```python
from build123d import *

# Parameters (mm, degrees)
F0_W     = 32
F0_H     = 32
F1_DEPTH = 600
F3_D     = 14
F3_DEPTH = 45
F4_D     = 14
F4_DEPTH = 45
F6_D     = 5
F6_DEPTH = 5
F7_D     = 5
F7_DEPTH = 5


with BuildPart() as f1:
    # F0 (on Front) → F1 (new body)
    with BuildSketch(Plane.XZ):
        with BuildLine():
            Line((-15, -20), (15, -20))
            ThreePointArc((15, -20), (18.535534, -18.535534), (20, -15))
            Line((20, -15), (20, 15))
            ThreePointArc((20, 15), (18.535534, 18.535534), (15, 20))
            Line((15, 20), (-15, 20))
            ThreePointArc((-15, 20), (-18.535534, 18.535534), (-20, 15))
            Line((-20, 15), (-20, -15))
            ThreePointArc((-20, -15), (-18.535534, -18.535534), (-15, -20))
        make_face()
        Rectangle(F0_W, F0_H, mode=Mode.SUBTRACT)
    extrude(amount=F1_DEPTH)

    # F3
    with Locations(Plane.YZ.offset(20)):
        with Locations((-560, 0)):
            Hole(F3_D / 2, depth=F3_DEPTH)

    # F4
    with Locations(Plane.YZ.offset(20)):
        with Locations((-40, 0)):
            Hole(F4_D / 2, depth=F4_DEPTH)

    # F6
    with Locations(Plane(origin=(0, 0, -20), x_dir=(1, 0, 0), z_dir=(0, 0, -1))):
        with Locations((0, 525)):
            Hole(F6_D / 2, depth=F6_DEPTH)

    # F7
    with Locations(Plane(origin=(0, 0, -20), x_dir=(1, 0, 0), z_dir=(0, 0, -1))):
        with Locations((0, 75)):
            Hole(F7_D / 2, depth=F7_DEPTH)


solid = f1.part
```
Geometry check sheet. Reference: the model listing, model coordinates, mm. A direction names the side the tool comes from. Coordinates: 2 decimals unless noted, no trailing zeros. Order: outer loops, then holes, each group sorted by start corner. A loop starts at its lowest first (then second) coordinate and runs counter-clockwise, first axis right, second up. Notation, with made-up numbers: M 13.25,52.5 L 46.25,52.5 A14 ccw 46.25,61.5 Z; hole C 41.5,46.5 d3. An arc over 180 degrees is marked long. Answer as a JSON object with one key per item and string values.
Q1. Cross-section at A-A on y = -40. Record the cut outline in (x, z).
Results are:
{"outline": "M -20,-15 A5 ccw -15,-20 L 15,-20 A5 ccw 20,-15 L 20,-7 L 16,-7 L 16,-16 L -16,-16 L -16,-7 L -20,-7 Z; M -20,7 L -16,7 L -16,16 L 16,16 L 16,7 L 20,7 L 20,15 A5 ccw 15,20 L -15,20 A5 ccw -20,15 Z"}
Q2. Release check for a two-part mould opening along Z. For faces 1 (the flat face through (-18, 0, 0)), 2 (the flat face through (0, -296, -20)), 3 (the flat face through (0, -296, 20)), 4 (the cylindrical face through (-18.028, -566.677, 2.103)) record: released by +Z, released by -Z, zero draft, split by the parting line, or undercut.
Results are:
{"face 1": "zero draft", "face 2": "released by -Z", "face 3": "released by +Z", "face 4": "undercut"}
Q3. Scan lines: line 1 (Y direction, x = 0, z = -16.9); line 2 (Z direction, x = 10.5, y = -228). Record each from-to range of solid material in increasing order.
Results are:
{"line 1": "y = -600 to -527.5, -522.5 to -77.5, -72.5 to 0", "line 2": "z = -20 to -16, 16 to 20"}
Q4. Tool access check on faces 5 (the flat face through (0, -296, 16)), 6 (the cylindrical face through (17.972, -46.677, 2.103)). Record the directions out of +Z, -Z, +X, -X, +Y, -Y that give a thin tool (end or side, any length) a straight path to the whole face; none if there is none.
Results are:
{"face 5": "+Y, -Y", "face 6": "+X, -X"}
Q5. Cross-section at C-C on y = -238. Record the cut outline in (x, z), and give its area (3 significant figures).
Results are:
{"outline": "M -20,-15 A5 ccw -15,-20 L 15,-20 A5 ccw 20,-15 L 20,15 A5 ccw 15,20 L -15,20 A5 ccw -20,15 Z; hole M -16,-16 L 16,-16 L 16,16 L -16,16 Z", "area": "555 mm²"}
Q6. Cross-section at B-B on z = 0. Record the cut outline in (x, y).
Results are:
{"outline": "M -20,-600 L -16,-600 L -16,-567 L -20,-567 Z; M -20,-553 L -16,-553 L -16,-47 L -20,-47 Z; M -20,-33 L -16,-33 L -16,0 L -20,0 Z; M 16,-600 L 20,-600 L 20,-567 L 16,-567 Z; M 16,-553 L 20,-553 L 20,-47 L 16,-47 Z; M 16,-33 L 20,-33 L 20,0 L 16,0 Z"}
Q7. Depth check by flat-ended pin: pin 1 Ø5 at (x, z) = (12.5, 5.5) entering from +Y. Enter the tip coordinate at first touch or a pass-through.
Results are:
{"pin 1": "passes through"}
